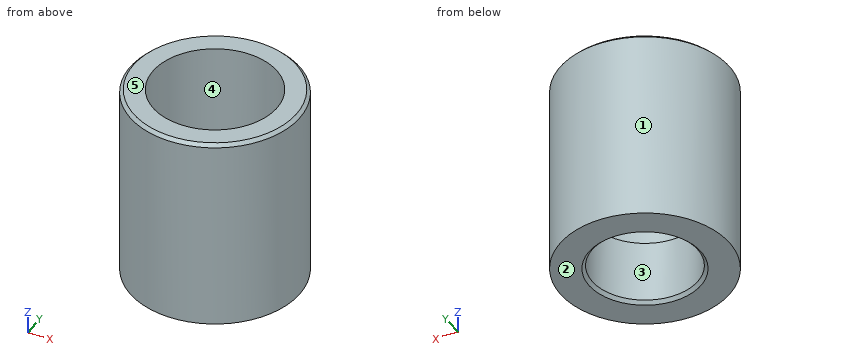
```python
from build123d import *

# Parameters (mm, degrees)
SKETCH_R        = 13
SKETCH_R_2      = 8.1
PAD_DEPTH       = 10
SKETCH001_R     = 13
SKETCH001_R_2   = 9.5
PAD001_DEPTH    = 20
CHAMFER_SIZE    = 0.5
CHAMFER001_SIZE = 0.5


with BuildPart() as part:
    # Sketch → Pad (new body)
    with BuildSketch(Plane.XY):
        Circle(SKETCH_R)
        Circle(SKETCH_R_2, mode=Mode.SUBTRACT)
    extrude(amount=PAD_DEPTH)

    # Sketch001 (on Face4 of Pad) → Pad001 (join)
    with BuildSketch(Plane.XY.offset(10)):
        Circle(SKETCH001_R)
        Circle(SKETCH001_R_2, mode=Mode.SUBTRACT)
    extrude(amount=PAD001_DEPTH)

    # Chamfer
    chamfer_edges = [part.edges().sort_by_distance(p)[0] for p in [
        (-8.1, 0, 0),
    ]]
    chamfer(chamfer_edges, length=CHAMFER_SIZE)

    # Chamfer001
    chamfer001_edges = [part.edges().sort_by_distance(p)[0] for p in [
        (-13, 0, 30),
    ]]
    chamfer(chamfer001_edges, length=CHAMFER001_SIZE)


solid = part.part
```
Geometry: final body of the model. Coordinates: model frame, mm. Face numbers are marked on the shaded views. A direction names the side the tool comes from. Give positions to 0.01 mm unless a question says otherwise; leave off trailing zeros. Loops run counter-clockwise (first coordinate to the right, second up) from the corner with the lowest first, then second, coordinate; pieces in that order, holes last. Notation, with made-up numbers: (-6.5, 60) -> (18.5, 60) arc R11 ccw to (18.5, 66) -> close; hole circle Ø5 at (-33.75, -15). An arc over 180 degrees is marked (long way). Return JSON: item names as keys, results as strings.
Item 1: Section C-C, the plane z = 14.5. Output: boundary loops of the cut face in (x, y), plus the area to 3 significant figures.
Filled in:
{"outline": "circle Ø26 at (0, 0); hole circle Ø19 at (0, 0)", "area": "247 mm^2"}
Item 2: Line query: line 1 (Y direction, x = 0, z = 7.5); line 2 (Y direction, x = 0, z = 20.5); line 3 (X direction, y = 6.75, z = 17.5). Output: solid intervals per line, ascending.
Filled in:
{"line 1": "-13 to -8.1, 8.1 to 13", "line 2": "-13 to -9.5, 9.5 to 13", "line 3": "-11.11 to -6.68, 6.68 to 11.11"}
Item 3: Access query for the marked faces 4 and 5. Directions: +Z, -Z, +X, -X, +Y, -Y. A direction counts if a zero-diameter tool reaches every point of the face in a straight line with its end or side. Return the directions, or none.
Filled in:
{"face 4": "+Z", "face 5": "+Z, +X, -X, +Y, -Y"}
Item 4: Section A-A, the plane x = 0. Output: boundary loops of the cut face in (y, z), plus the area to 4 significant figures.
Filled in:
{"outline": "(-13, 0) -> (-8.6, 0) -> (-8.1, 0.5) -> (-8.1, 10) -> (-9.5, 10) -> (-9.5, 30) -> (-12.5, 30) -> (-13, 29.5) -> close; (8.1, 0.5) -> (8.6, 0) -> (13, 0) -> (13, 29.5) -> (12.5, 30) -> (9.5, 30) -> (9.5, 10) -> (8.1, 10) -> close", "area": "237.5 mm^2"}
Item 5: Pin query (flat end, axial travel): P1, Ø5, axis at y = 8, z = 7.5, coming from the -X side; P2, Ø6, axis at x = -9.5, z = 15.5, coming from the +Y side; P3, Ø13, axis at x = 0, y = 0, coming from the +Z side; P4, Ø5.5, axis at x = -3.5, y = 4.5, coming from the +Z side. Return the tip coordinate at first contact, or that it passes through.
Filled in:
{"P1": "x = -11.78", "P2": "y = 11.26", "P3": "through", "P4": "z = 10"}
Item 6: Mould query, pull axis X, two halves, no side actions, for the marked faces 1, 2 and 3. Classes: released by +X, released by -X, zero draft, split by the parting line, or undercut.
Filled in:
{"face 1": "split by the parting line", "face 2": "zero draft", "face 3": "undercut"}
